```python
from build123d import *

# Parameters (mm, degrees)
TAP_DRILL_FOR_M4X0_7_TAP1_D = 3.3
CUT_EXTRUDE1_DEPTH          = 10.165790389
CUT_EXTRUDE1_DEPTH_BACK     = 10.165790389
SKETCH5_W                   = 1
SKETCH5_H                   = 3.627718677


with BuildPart() as part:
    # Sketch1 → Revolve1 (revolve)
    with BuildSketch(Plane.XY, mode=Mode.PRIVATE) as revolve1_sk:
        with BuildLine():
            Line((0, 0), (0, 8.127718677))
            ThreePointArc((0, 8.127718677), (2.474873734, 7.102592411), (3.5, 4.627718677))
            Line((3.5, 4.627718677), (3.5, 0))
            Line((3.5, 0), (0, 0))
        make_face()
    revolve(revolve1_sk.sketch.rotate(Axis((0, 8.127718677, 0), (0, 1, 0)), 90), axis=Axis((0, 8.127718677, 0), (0, 1, 0)))

    # Tap Drill for M4x0.7 Tap1 (through all)
    with Locations(Plane(origin=(0, 0, 0), x_dir=(-1, 0, 0), z_dir=(0, -1, 0))):
        with Locations((0, 0)):
            Hole(TAP_DRILL_FOR_M4X0_7_TAP1_D / 2)

    # Sketch5 → Cut-Extrude1 (cut, two sides: drawn at the far end of the back side and taken through both)
    with BuildSketch(Plane.XY.offset(-CUT_EXTRUDE1_DEPTH_BACK)):
        with Locations((3, 2.313859338)):
            Rectangle(SKETCH5_W, SKETCH5_H)
        with Locations((-3, 2.313859338)):
            Rectangle(SKETCH5_W, SKETCH5_H)
    extrude(amount=CUT_EXTRUDE1_DEPTH + CUT_EXTRUDE1_DEPTH_BACK, mode=Mode.SUBTRACT)


solid = part.part
```
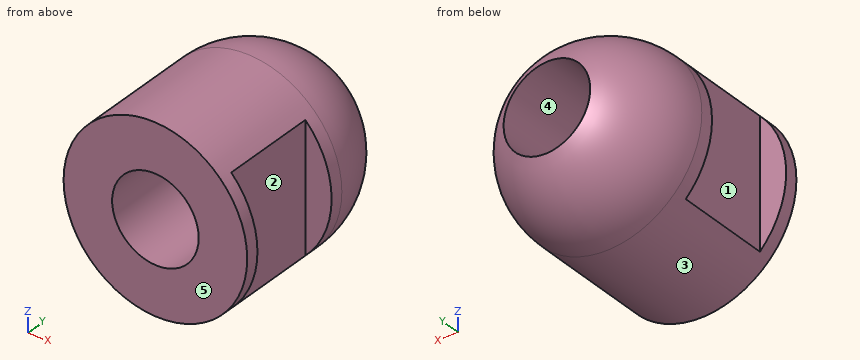
The listing builds one solid part. Answer for the finished solid, in the listing's coordinates (mm). Face numbers are marked on the shaded views. A direction names the side the tool comes from. Round coordinates to 2 decimals unless told otherwise and drop trailing zeros. Loops run counter-clockwise (first coordinate to the right, second up) from the corner with the lowest first, then second, coordinate; pieces in that order, holes last. Notation, with made-up numbers: (80, 18.5) -> (113, 18.5) arc R22 cw to (113, 35.5) -> close; hole circle Ø11 at (57, 42.5). An arc over 180 degrees is marked (long way). Use one line per item in the form item = value.
1. Find the intervals of material crossed by probe 1 along X at (y, z) = (4, 0.25); probe 2 along X at (y, z) = (7, 1.25); probe 3 along Z at (x, y) = (-0.25, 4), in increasing order. Write a range as [from, to].
Answer key:
probe_1 = [-2.5, -1.63], [1.63, 2.5]
probe_2 = [-2.25, -1.08], [1.08, 2.25]
probe_3 = [-3.49, -1.63], [1.63, 3.49]
2. The part is cut by section C-C on z = -2.25. Determine the outline of the cut face in (x, y), and give its area (3 significant figures).
Answer key:
outline = (-2.68, 0) -> (2.68, 0) -> (2.68, 0.5) -> (2.5, 0.5) -> (2.5, 4.13) -> (2.68, 4.13) -> (2.68, 4.63) arc R2.68 ccw to (-2.68, 4.63) -> (-2.68, 4.13) -> (-2.5, 4.13) -> (-2.5, 0.5) -> (-2.68, 0.5) -> close
area = 34.8 mm²
3. For a pull along Z with two mould halves and no side action, classify the marked faces 3, 4 and 5 as released by +Z, released by -Z, zero draft, split by the parting line, or undercut.
Answer key:
face_3 = split by the parting line
face_4 = undercut
face_5 = zero draft
4. The part is cut by section D-D on x = 1.25. Determine the outline of the cut face in (y, z).
Answer key:
outline = (0, -3.27) -> (4.63, -3.27) arc R3.27 ccw to (7.71, -1.08) -> (0, -1.08) -> close; (0, 1.08) -> (7.71, 1.08) arc R3.27 ccw to (4.63, 3.27) -> (0, 3.27) -> close
5. The part is cut by section A-A on x = 0. Determine the outline of the cut face in (y, z).
Answer key:
outline = (0, -3.5) -> (4.63, -3.5) arc R3.5 ccw to (7.71, -1.65) -> (0, -1.65) -> close; (0, 1.65) -> (7.71, 1.65) arc R3.5 ccw to (4.63, 3.5) -> (0, 3.5) -> close
6. Flat-ended cylindrical pins translate along their axes: pin 1 Ø1.8 at (y, z) = (1.5, 1) entering from -X; pin 2 Ø0.5 at (x, z) = (3, -0.5) entering from +Y; pin 3 Ø1.1 at (x, z) = (-3, -0.5) entering from +Y; pin 4 Ø2 at (x, z) = (0, 0) entering from -Y. Find the tip coordinate at first contact, or state that the pin passes through.
Answer key:
pin_1 = -2.5
pin_2 = 6.74
pin_3 = 7.09
pin_4 = through
7. A tool of negligible diameter and unlimited length cuts with its end or side. For the marked faces 1 and 2, from which of +Z, -Z, +X, -X, +Y, -Y can it reach the whole face along a straight path? Write none if from no direction.
Answer key:
face_1 = +Z, -Z, -X
face_2 = +Z, -Z, +X
8. The part is cut by section B-B on y = 2.5. Determine the outline of the cut face in (x, z).
Answer key:
outline = (-2.5, -2.45) arc R3.5 ccw to (2.5, -2.45) -> (2.5, 2.45) arc R3.5 ccw to (-2.5, 2.45) -> close; hole circle Ø3.3 at (0, 0)
